from build123d import *

# Parameters (mm, degrees)
IZIM1_W               = 160
IZIM1_H               = 210
TABAN_FLAN_1_DEPTH    = 8
K_ELERI_START         = -8
K_ELERI_K_R1_DEPTH    = 8
IZIM6_R               = 8.5
KES_EKSTR_ZYON1_DEPTH = 10


# Read off the part's stored shape, not the designer's step: Köşeleri kır1
# Sheet-metal steps are written as plain solids
with BuildPart() as part:
    # Çizim1 → Taban-Flanş1 (new body)
    with BuildSketch(Plane(origin=(0, 0, 0), x_dir=(1, 0, 0), z_dir=(0, 1, 0))):
        with Locations((0, 105)):
            Rectangle(IZIM1_W, IZIM1_H)
    extrude(amount=-TABAN_FLAN_1_DEPTH)

    # Köşeleri kır1 outline → Köşeleri kır1 (cut)
    with BuildSketch(Plane(origin=(0, 0, 0), x_dir=(1, 0, 0), z_dir=(0, 1, 0)).offset(K_ELERI_START)):
        with BuildLine():
            ThreePointArc((-80, 206), (-78.828427125, 208.828427125), (-76, 210))
            Line((-76, 210), (-80, 210))
            Line((-80, 210), (-80, 206))
        make_face()
        with BuildLine():
            Line((80, 210), (76, 210))
            ThreePointArc((76, 210), (78.828427125, 208.828427125), (80, 206))
            Line((80, 206), (80, 210))
        make_face()
        with BuildLine():
            ThreePointArc((-76, 0), (-78.828427125, 1.171572875), (-80, 4))
            Line((-80, 4), (-80, 0))
            Line((-80, 0), (-76, 0))
        make_face()
        with BuildLine():
            Line((80, 0), (80, 4))
            ThreePointArc((80, 4), (78.828427125, 1.171572875), (76, 0))
            Line((76, 0), (80, 0))
        make_face()
    extrude(amount=K_ELERI_K_R1_DEPTH, mode=Mode.SUBTRACT)

    # Çizim6 → Kes-Ekstrüzyon1 (cut)
    with BuildSketch(Plane(origin=(0, 0, 0), x_dir=(1, 0, 0), z_dir=(0, 1, 0))):
        with Locations(Location((0, 72, 0), (0, 0, 270))):
            Circle(IZIM6_R)
    extrude(amount=-KES_EKSTR_ZYON1_DEPTH, mode=Mode.SUBTRACT)


solid = part.part
Model file for the job. Use its own axes, mm. Round coordinates to 2 decimals unless told otherwise and drop trailing zeros. Loops run counter-clockwise (first coordinate to the right, second up) from the corner with the lowest first, then second, coordinate; pieces in that order, holes last. Notation, with made-up numbers: (18, -37.5) - (70, -37.5) arc R21 cw to (70, -14.5) - close; hole circle Ø8 at (-9, 6.5). An arc over 180 degrees is marked (long way). Write each question's results on one line, items separated by ' | '.
(1) Wall check: L1, parallel to X at y = -4.5, z = -72; L2, parallel to Z at x = 6, y = -2.5; L3, parallel to Z at x = 6.5, y = -4. Give the ranges that are in metal, low to high.
Answer below:
L1: x = -80 to -8.5, 8.5 to 80 | L2: z = -210 to -78.02, -65.98 to 0 | L3: z = -210 to -77.48, -66.52 to 0
(2) Saw through at A-A, the plane z = -72. List the corners of the cut face in (x, y).
Answer below:
outline: (-80, -8) - (-8.5, -8) - (-8.5, 0) - (-80, 0) - close; (8.5, -8) - (80, -8) - (80, 0) - (8.5, 0) - close
(3) Pin check, flat tip, straight feed: pin 1 (12 mm diameter, centred on x = -50.5, z = -102.5, fed in from +Y). Stop position of the tip, or through.
Answer below:
pin 1: stops at y = 0
(4) Saw through at B-B, the plane x = 0. List the corners of the cut face in (y, z).
Answer below:
outline: (-8, -210) - (0, -210) - (0, -80.5) - (-8, -80.5) - close; (-8, -63.5) - (0, -63.5) - (0, 0) - (-8, 0) - close
